CAD build for the part. Positions are in the model's coordinates, mm. A direction names the side the tool comes from. Coordinates: 2 decimals unless noted, no trailing zeros. Write each loop counter-clockwise with the first axis right and the second up, starting at its lowest first coordinate (ties: lowest second). Pieces come first, ordered by that corner, then holes.
```python
from build123d import *

# Parameters (mm, degrees)
BOSS_EXTRU_1_DEPTH      = 15
ESQUISSE2_R             = 3.5
ENL_V_MAT_EXTRU_1_DEPTH = 4
ESQUISSE5_R             = 1.75
ENL_V_MAT_EXTRU_2_DEPTH = 20


with BuildPart() as part:
    # Esquisse1 → Boss.-Extru.1 (new body)
    with BuildSketch(Plane.XY):
        with BuildLine():
            Line((8.142533049, 9), (8.142533049, 19))
            Line((8.142533049, 19), (-5.354330929, 19))
            Line((-5.354330929, 19), (-5.354330929, 10.929236708))
            ThreePointArc((-5.354330929, 10.929236708), (4.975752737, 5.769164862), (9.142533049, -5))
            ThreePointArc((9.142533049, -5), (-17.628961192, -16.83109935), (-8.354330929, 10.929827313))
            Line((-8.354330929, 10.929827313), (-8.354330929, 19))
            Line((-8.354330929, 19), (-25.857466951, 19))
            Line((-25.857466951, 19), (-25.857466951, -29))
            Line((-25.857466951, -29), (12.142533049, -29))
            Line((12.142533049, -29), (12.142533049, 9))
            Line((12.142533049, 9), (8.142533049, 9))
        make_face()
    extrude(amount=BOSS_EXTRU_1_DEPTH)

    # Esquisse2 → Enlèv. mat.-Extru.1 (cut)
    with BuildSketch(Plane(origin=(8.142533049, 0, 0), x_dir=(0, 0, -1), z_dir=(1, 0, 0))):
        with Locations((-7.5, 14)):
            Circle(ESQUISSE2_R)
    extrude(amount=-ENL_V_MAT_EXTRU_1_DEPTH, mode=Mode.SUBTRACT)

    # Esquisse5 → Enlèv. mat.-Extru.2 (cut)
    with BuildSketch(Plane(origin=(4.142533049, 0, 0), x_dir=(0, 0, -1), z_dir=(1, 0, 0))):
        with Locations((-7.5, 14)):
            Circle(ESQUISSE5_R)
    extrude(amount=-ENL_V_MAT_EXTRU_2_DEPTH, mode=Mode.SUBTRACT)


solid = part.part
```
Item 1: Saw through at D-D, the plane y = -11.5. Write the cut outline in (x, z).
Item 2: Two-plate mould, pull along Y, no slides. Class faces 1 (the flat face through (1, 19, 7)), 2 (the flat face through (4.143, 16, 7)), 3 (the flat face through (8.143, 10.6, 5.7)): +Y half, -Y half, draft (parallel to the pull), parting line (faces both ways), or undercut.
Item 3: Saw through at C-C, the plane z = 7.5. Write the cut outline in (x, y).
Item 4: Saw through at A-A, the plane y = 14. Write the cut outline in (x, z).
Item 5: Flat gauge pins, fed straight in: pin 1 Ø4.5 at (y, z) = (14, 7.5) entering from +X; pin 2 Ø3 at (y, z) = (14, 7.5) entering from +X; pin 3 Ø4 at (y, z) = (15.5, 9.5) entering from +X. Where does each tip first touch, or does it go through?
Item 6: Saw through at B-B, the plane x = -2. Write the cut outline in (y, z).
Item 7: Which spindle directions (+Z, -Z, +X, -X, +Y, -Y) get a long thin tool onto all of the face, cutting with end or side? Do faces 4 (the flat face through (12.143, -10, 7)), 5 (the cylindrical face through (-0.539, 15.735, 7.728)), 6 (the flat face through (10, 9, 7)), 7 (the flat face through (-8.354, 16, 7)), 8 (the flat face through (-11, -21, 15)). Say none if no direction does.
Item 8: Wall check: line 1 along X through (y, z) = (12.5, 10.25); line 2 along Y through (x, z) = (-12.75, 7.5); line 3 along X through (y, z) = (-3.5, 1.5). Give the ranges that are in metal, low to high.
Working result:
1. outline: (-25.86, 0) - (-21.48, 0) - (-21.48, 15) - (-25.86, 15) - close; (7.76, 0) - (12.14, 0) - (12.14, 15) - (7.76, 15) - close
2. face 1: +Y half
2. face 2: undercut
2. face 3: draft
3. outline: (-25.86, -29) - (12.14, -29) - (12.14, 9) - (8.14, 9) - (8.14, 10.5) - (4.14, 10.5) - (4.14, 12.25) - (-5.35, 12.25) - (-5.35, 10.93) arc R16 cw (long way) to (-8.35, 10.93) - (-8.35, 12.25) - (-15.86, 12.25) - (-15.86, 15.75) - (-8.35, 15.75) - (-8.35, 19) - (-25.86, 19) - close; (-5.35, 15.75) - (4.14, 15.75) - (4.14, 17.5) - (8.14, 17.5) - (8.14, 19) - (-5.35, 19) - close
4. outline: (-25.86, 0) - (-8.35, 0) - (-8.35, 5.75) - (-15.86, 5.75) - (-15.86, 9.25) - (-8.35, 9.25) - (-8.35, 15) - (-25.86, 15) - close; (-5.35, 0) - (8.14, 0) - (8.14, 4) - (4.14, 4) - (4.14, 5.75) - (-5.35, 5.75) - close; (-5.35, 9.25) - (4.14, 9.25) - (4.14, 11) - (8.14, 11) - (8.14, 15) - (-5.35, 15) - close
5. pin 1: stops at x = 4.14
5. pin 2: stops at x = -15.86
5. pin 3: stops at x = 8.14
6. outline: (-29, 0) - (-20.24, 0) - (-20.24, 15) - (-29, 15) - close; (10.24, 0) - (19, 0) - (19, 15) - (10.24, 15) - close; hole circle Ø3.5 at (14, 7.5)
7. face 4: +Z, -Z, +X, +Y, -Y
7. face 5: +X
7. face 6: +Z, -Z, +X, +Y
7. face 7: +Z, -Z, +Y
7. face 8: +Z, +X, -X, +Y, -Y
8. line 1: x = -25.86 to -8.35, -5.35 to 4.14
8. line 2: y = -29 to -19.88, 9.88 to 12.25, 15.75 to 19
8. line 3: x = -25.86 to -22.79, 9.07 to 12.14
